from build123d import *

# Parameters (mm, degrees)
BOSS_EXTRUDE1_DEPTH = 10
CHAMFER1_SIZE       = 10
SKETCH2_R           = 6
CUT_EXTRUDE1_DEPTH  = 10
SKETCH3_R           = 6
CUT_EXTRUDE2_DEPTH  = 10


with BuildPart() as part:
    # Sketch1 → Boss-Extrude1 (new, symmetric)
    with BuildSketch(Plane(origin=(0, 0, 0), x_dir=(1, 0, 0), z_dir=(0, 1, 0))):
        with BuildLine():
            Line((-32.5, 62.5), (32.5, 62.5))
            ThreePointArc((32.5, 62.5), (53.713203436, 53.713203436), (62.5, 32.5))
            Line((62.5, 32.5), (62.5, -32.5))
            ThreePointArc((62.5, -32.5), (53.713203436, -53.713203436), (32.5, -62.5))
            Line((32.5, -62.5), (-32.5, -62.5))
            ThreePointArc((-32.5, -62.5), (-53.713203436, -53.713203436), (-62.5, -32.5))
            Line((-62.5, -32.5), (-62.5, 32.5))
            ThreePointArc((-62.5, 32.5), (-53.713203436, 53.713203436), (-32.5, 62.5))
        make_face()
    extrude(amount=BOSS_EXTRUDE1_DEPTH, both=True)

    # Chamfer1
    chamfer1_edges = [part.edges().sort_by_distance(p)[0] for p in [
        (53.713203436, 10, 53.713203436),
        (62.5, 10, 0),
        (53.713203436, 10, -53.713203436),
        (0, 10, -62.5),
        (-53.713203436, 10, -53.713203436),
        (-62.5, 10, 0),
        (-53.713203436, 10, 53.713203436),
        (0, 10, 62.5),
    ]]
    chamfer(chamfer1_edges, length=CHAMFER1_SIZE)

    # Sketch2 → Cut-Extrude1 (cut)
    with BuildSketch(Plane(origin=(0, 10, 0), x_dir=(1, 0, 0), z_dir=(0, 1, 0))):
        with Locations(Location((12.5, 12.5, 0), (0, 0, 270))):
            Circle(SKETCH2_R)
        with Locations(Location((-12.5, 12.5, 0), (0, 0, 90))):
            Circle(SKETCH2_R)
        with Locations(Location((12.5, -12.5, 0), (0, 0, 90))):
            Circle(SKETCH2_R)
        with Locations(Location((-12.5, -12.5, 0), (0, 0, 270))):
            Circle(SKETCH2_R)
    extrude(amount=-CUT_EXTRUDE1_DEPTH, mode=Mode.SUBTRACT)

    # Sketch3 → Cut-Extrude2 (cut)
    with BuildSketch(Plane.XZ.offset(10)):
        with Locations(Location((37.5, 37.5, 0), (0, 0, 270))):
            Circle(SKETCH3_R)
        with Locations(Location((-37.5, 37.5, 0), (0, 0, 270))):
            Circle(SKETCH3_R)
        with Locations(Location((37.5, -37.5, 0), (0, 0, 270))):
            Circle(SKETCH3_R)
        with Locations(Location((-37.5, -37.5, 0), (0, 0, 270))):
            Circle(SKETCH3_R)
    extrude(amount=-CUT_EXTRUDE2_DEPTH, mode=Mode.SUBTRACT)


solid = part.part
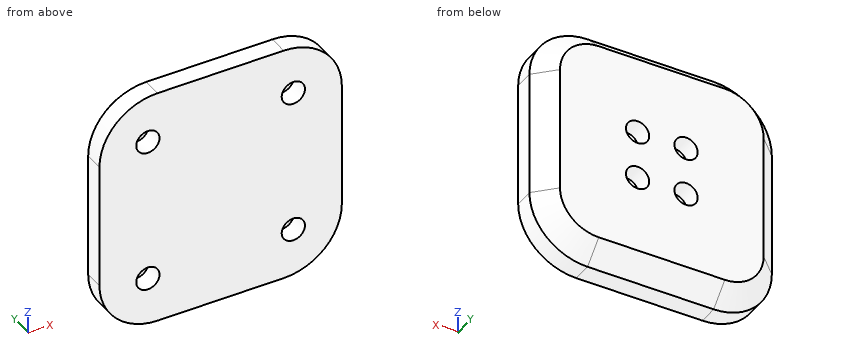
Could you check a few things on this model? Use its own coordinates, in mm. Coordinates: 2 decimals unless noted, no trailing zeros. Order: outer loops, then holes, each group sorted by start corner. A loop starts at its lowest first (then second) coordinate and runs counter-clockwise, first axis right, second up.
Q1. Will these pins go through, and if not, where does the flat tip stop? pin 1 (13 mm diameter, centred on x = 39, z = -38, fed in from -Y); pin 2 (3.5 mm diameter, centred on x = -36.5, z = -40, fed in from -Y); pin 3 (3.5 mm diameter, centred on x = 10.5, z = -14.5, fed in from +Y); pin 4 (1.5 mm diameter, centred on x = 38.5, y = 7, fed in from -Z).
Q2. Suppose I cut it at C-C on x = 12.5. Please give me the cut outline in (y, z).
Q3. Please list where these lines run through material, in increasing order: L1, parallel to X at y = -5.25, z = 37.5; L2, parallel to X at y = 8, z = -12.5; L3, parallel to Z at x = -16, y = 0.5.
Q4. Suppose I cut it at D-D on z = -26.5. Please give me the cut outline in (x, y).
Q5. Suppose I cut it at A-A on y = 3.25. Please give me the cut outline in (x, z), and give its area (3 significant figures).
Q6. Suppose I cut it at B-B on z = 12.5. Please give me the cut outline in (x, y), and give its area (3 significant figures).
Answer:
1. pin 1: stops at y = -10
1. pin 2: stops at y = 0
1. pin 3: stops at y = 0
1. pin 4: stops at z = -55.5
2. outline: (-10, -62.5) - (0, -62.5) - (10, -52.5) - (10, -18.5) - (0, -18.5) - (0, -6.5) - (10, -6.5) - (10, 6.5) - (0, 6.5) - (0, 18.5) - (10, 18.5) - (10, 52.5) - (0, 62.5) - (-10, 62.5) - close
3. L1: x = -62.08 to -43.5, -31.5 to 31.5, 43.5 to 62.08
3. L2: x = -54.5 to -18.5, -6.5 to 6.5, 18.5 to 54.5
3. L3: z = -62 to -17.37, -7.63 to 7.63, 17.37 to 62
4. outline: (-62.5, -10) - (62.5, -10) - (62.5, 0) - (52.5, 10) - (-52.5, 10) - (-62.5, 0) - close
5. outline: (-59.25, -32.5) arc R26.75 ccw to (-32.5, -59.25) - (32.5, -59.25) arc R26.75 ccw to (59.25, -32.5) - (59.25, 32.5) arc R26.75 ccw to (32.5, 59.25) - (-32.5, 59.25) arc R26.75 ccw to (-59.25, 32.5) - close; hole circle Ø12 at (-12.5, -12.5); hole circle Ø12 at (-12.5, 12.5); hole circle Ø12 at (12.5, -12.5); hole circle Ø12 at (12.5, 12.5)
5. area: 13,000 mm2
6. outline: (-62.5, -10) - (62.5, -10) - (62.5, 0) - (52.5, 10) - (18.5, 10) - (18.5, 0) - (6.5, 0) - (6.5, 10) - (-6.5, 10) - (-6.5, 0) - (-18.5, 0) - (-18.5, 10) - (-52.5, 10) - (-62.5, 0) - close
6. area: 2,160 mm2
